from build123d import *

# Parameters (mm, degrees)
F0_R     = 4.1
F1_DEPTH = 3.4
F0_R_2   = 3.8
F0_R_3   = 1.95
F2_DEPTH = 3.72
F3_DEPTH = 3.28
F4_SIZE  = 0.1
F5_SIZE  = 0.1
F6_SIZE  = 0.1
F7_DEPTH = 3.72


# Not quite as in the source:
# - a feature names something its author has since deleted; it is built from what else it names


with BuildPart() as f1:
    # F0 (on Front) → F1 (new body)
    with BuildSketch(Plane.XZ):
        with BuildLine():
            ThreePointArc((-9.1306946704, 2.3368867827), (-8.1937279785, 1.5734002793), (-7.0529357563, 1.1741367966))
            ThreePointArc((-7.0529357563, 1.1741367966), (-7.1195743604, 0.6589088915), (-7.1486252748, 0.1402022865))
            ThreePointArc((-7.1486252748, 0.1402022865), (-8.3432287104, -0.042236429), (-9.4045806012, -0.6200715414))
            ThreePointArc((-9.4045806012, -0.6200715414), (-9.3954740629, -0.7454476061), (-9.384696163, -0.870691063))
            ThreePointArc((-9.384696163, -0.870691063), (-9.3722488189, -0.9957796327), (-9.3581342447, -1.120691063))
            ThreePointArc((-9.3581342447, -1.120691063), (-8.2085925976, -1.4934044314), (-7.0008156513, -1.4529556828))
            ThreePointArc((-7.0008156513, -1.4529556828), (-6.8768331336, -1.9574641892), (-6.7165444751, -2.4516382918))
            ThreePointArc((-6.7165444751, -2.4516382918), (-7.76441436, -3.053950319), (-8.544935067, -3.9767712658))
            ThreePointArc((-8.544935067, -3.9767712658), (-8.4914364249, -4.0897594601), (-8.43644384, -4.2020281216))
            ThreePointArc((-8.43644384, -4.2020281216), (-8.3799669873, -4.3135574983), (-8.3220158032, -4.4243279682))
            ThreePointArc((-8.3220158032, -4.4243279682), (-7.1152349462, -4.3573127689), (-6.0032028311, -3.8838197394))
            ThreePointArc((-6.0032028311, -3.8838197394), (-5.7053436074, -4.3094726268), (-5.3773631048, -4.7123737159))
            ThreePointArc((-5.3773631048, -4.7123737159), (-6.1368874979, -5.6525550384), (-6.5313316874, -6.7950225452))
            ThreePointArc((-6.5313316874, -6.7950225452), (-6.4406375804, -6.8810473446), (-6.3488105376, -6.9658617383))
            ThreePointArc((-6.3488105376, -6.9658617383), (-6.255866712, -7.0494508071), (-6.1618224526, -7.1317998474))
            ThreePointArc((-6.1618224526, -7.1317998474), (-5.0607335264, -6.6333809478), (-4.1948295471, -5.7901558762))
            ThreePointArc((-4.1948295471, -5.7901558762), (-3.7633208909, -6.0794667424), (-3.3119438366, -6.3366811521))
            ThreePointArc((-3.3119438366, -6.3366811521), (-3.6805479914, -7.487745529), (-3.6356508664, -8.6955544836))
            ThreePointArc((-3.6356508664, -8.6955544836), (-3.5200054468, -8.7430078723), (-3.4037408432, -8.7889233284))
            ThreePointArc((-3.4037408432, -8.7889233284), (-3.2868775071, -8.8332927753), (-3.1694359951, -8.8761084081))
            ThreePointArc((-3.1694359951, -8.8761084081), (-2.3227497605, -8.0135884705), (-1.8199250223, -6.9145045313))
            ThreePointArc((-1.8199250223, -6.9145045313), (-1.3130441845, -7.0284005982), (-0.7992311491, -7.1051903261))
            ThreePointArc((-0.7992311491, -7.1051903261), (-0.727143962, -8.311678782), (-0.2489808346, -9.4217107546))
            ThreePointArc((-0.2489808346, -9.4217107546), (-0.123991383, -9.4241843752), (0.0010198831, -9.4249999448))
            ThreePointArc((0.0010198831, -9.4249999448), (0.1260309698, -9.4241573201), (0.2510198831, -9.4216566494))
            ThreePointArc((0.2510198831, -9.4216566494), (0.7289427654, -8.3115212183), (0.8007688415, -7.1050171895))
            ThreePointArc((0.8007688415, -7.1050171895), (1.3145652461, -7.0281162635), (1.8214214224, -6.9141104997))
            ThreePointArc((1.8214214224, -6.9141104997), (2.3244840135, -8.0130855914), (3.1713568956, -8.8754222683))
            ThreePointArc((3.1713568956, -8.8754222683), (3.2887891386, -8.8325812196), (3.4056428696, -8.7881864821))
            ThreePointArc((3.4056428696, -8.7881864821), (3.5218975334, -8.742245865), (3.6375326803, -8.6947674494))
            ThreePointArc((3.6375326803, -8.6947674494), (3.6821684093, -7.4869488064), (3.3133151488, -6.3359642301))
            ThreePointArc((3.3133151488, -6.3359642301), (3.764636526, -6.078652139), (4.1960825592, -5.7892478921))
            ThreePointArc((4.1960825592, -5.7892478921), (5.0621690097, -6.6322855443), (6.1633657783, -7.1304661337))
            ThreePointArc((6.1633657783, -7.1304661337), (6.2573922134, -7.0480967422), (6.3503179465, -6.9644875604))
            ThreePointArc((6.3503179465, -6.9644875604), (6.4421266315, -6.8796532953), (6.5328021188, -6.7936088699))
            ThreePointArc((6.5328021188, -6.7936088699), (6.1381106848, -5.6512267557), (5.3783828347, -4.7112098322))
            ThreePointArc((5.3783828347, -4.7112098322), (5.7062761334, -4.3082377707), (6.00404323, -3.8825204303))
            ThreePointArc((6.00404323, -3.8825204303), (7.1161845365, -4.3557644871), (8.3229834462, -4.4225073832))
            ThreePointArc((8.3229834462, -4.4225073832), (8.3809053661, -4.3117340184), (8.4373530488, -4.2002022011))
            ThreePointArc((8.4373530488, -4.2002022011), (8.492316565, -4.0879315502), (8.5457862464, -3.9749418147))
            ThreePointArc((8.5457862464, -3.9749418147), (7.7650725635, -3.0522802473), (6.7170749034, -2.4501846343))
            ThreePointArc((6.7170749034, -2.4501846343), (6.8772566086, -1.9559758535), (7.0011299372, -1.4514405265))
            ThreePointArc((7.0011299372, -1.4514405265), (8.2090091905, -1.4913388042), (9.3584507476, -1.1180449923))
            ThreePointArc((9.3584507476, -1.1180449923), (9.3724970598, -0.9934404183), (9.3848843789, -0.868659999))
            ThreePointArc((9.3848843789, -0.868659999), (9.3956105125, -0.7437258211), (9.4046735619, -0.618659999))
            ThreePointArc((9.4046735619, -0.618659999), (8.3432765874, -0.0407321266), (7.1485947646, 0.1417493946))
            ThreePointArc((7.1485947646, 0.1417493946), (7.119431592, 0.6604497002), (7.0526814835, 1.1756631713))
            ThreePointArc((7.0526814835, 1.1756631713), (8.19338727, 1.5751735359), (9.1301887056, 2.3388628005))
            ThreePointArc((9.1301887056, 2.3388628005), (9.0983662855, 2.4597471284), (9.0649434237, 2.5801987762))
            ThreePointArc((9.0649434237, 2.5801987762), (9.0299259996, 2.7001965561), (8.9933201729, 2.8197193598))
            ThreePointArc((8.9933201729, 2.8197193598), (7.794773105, 2.9756140317), (6.6146636541, 2.7145395084))
            ThreePointArc((6.6146636541, 2.7145395084), (6.4000942258, 3.1876784501), (6.1517355927, 3.6439880896))
            ThreePointArc((6.1517355927, 3.6439880896), (7.0710932374, 4.4285897362), (7.6687594725, 5.4791197426))
            ThreePointArc((7.6687594725, 5.4791197426), (7.5954176181, 5.5803455276), (7.5207396972, 5.6805897059))
            ThreePointArc((7.5207396972, 5.6805897059), (7.444738846, 5.7798346442), (7.3674284334, 5.8780628849))
            ThreePointArc((7.3674284334, 5.8780628849), (6.1935005716, 5.5904666436), (5.1873914517, 4.9207184361))
            ThreePointArc((5.1873914517, 4.9207184361), (4.8163943669, 5.2843963991), (4.4199691978, 5.6201754679))
            ThreePointArc((4.4199691978, 5.6201754679), (4.9938151748, 6.683904295), (5.1716286044, 7.8793960795))
            ThreePointArc((5.1716286044, 7.8793960795), (5.0666724743, 7.9472923086), (4.9608250949, 8.0137905749))
            ThreePointArc((4.9608250949, 8.0137905749), (4.8541050851, 8.0788791811), (4.7465312174, 8.1425466779))
            ThreePointArc((4.7465312174, 8.1425466779), (3.7557669795, 7.4503007335), (3.0595379066, 6.4623314522))
            ThreePointArc((3.0595379066, 6.4623314522), (2.5822180472, 6.6674320361), (2.0912654051, 6.8373320093))
            ThreePointArc((2.0912654051, 6.8373320093), (2.2421089696, 8.0365222748), (1.9760667465, 9.2155187165))
            ThreePointArc((1.9760667465, 9.2155187165), (1.8536604305, 9.2409181367), (1.7309279903, 9.2646917538))
            ThreePointArc((1.7309279903, 9.2646917538), (1.6078910188, 9.2868353852), (1.4845711627, 9.307345135))
            ThreePointArc((1.4845711627, 9.307345135), (0.8107889051, 8.3039366723), (0.5184795371, 7.1311765488))
            ThreePointArc((0.5184795371, 7.1311765488), (-0.0006988298, 7.1499999658), (-0.5198735073, 7.1310750618))
            ThreePointArc((-0.5198735073, 7.1310750618), (-0.8124228005, 8.3037784061), (-1.4864122256, 9.307051289))
            ThreePointArc((-1.4864122256, 9.307051289), (-1.609717186, 9.2865190239), (-1.7327389902, 9.2643532204))
            ThreePointArc((-1.7327389902, 9.2643532204), (-1.8554559982, 9.2405577775), (-1.9778466235, 9.2151368809))
            ThreePointArc((-1.9778466235, 9.2151368809), (-2.2436700583, 8.0360880591), (-2.0926019054, 6.8369230846))
            ThreePointArc((-2.0926019054, 6.8369230846), (-2.5835911424, 6.6669000899), (-3.0609364181, 6.4616691531))
            ThreePointArc((-3.0609364181, 6.4616691531), (-3.7573792917, 7.4494877329), (-4.7482933229, 8.141519239))
            ThreePointArc((-4.7482933229, 8.141519239), (-4.8558534091, 8.0778284625), (-4.9625593299, 8.0127167613))
            ThreePointArc((-4.9625593299, 8.0127167613), (-5.0683923152, 7.946195589), (-5.1733337487, 7.8782766469))
            ThreePointArc((-5.1733337487, 7.8782766469), (-4.9952615939, 6.6828233728), (-4.4211854174, 5.6192187629))
            ThreePointArc((-4.4211854174, 5.6192187629), (-4.8175379075, 5.2833539073), (-5.1884562761, 4.9195956613))
            ThreePointArc((-5.1884562761, 4.9195956613), (-6.19471032, 5.5891261102), (-7.3687003961, 5.8764682823))
            ThreePointArc((-7.3687003961, 5.8764682823), (-7.4459895483, 5.7782233123), (-7.521968919, 5.6789619282))
            ThreePointArc((-7.521968919, 5.6789619282), (-7.5966251432, 5.5787015903), (-7.6699450885, 5.477459935))
            ThreePointArc((-7.6699450885, 5.477459935), (-7.0720515108, 4.4270593007), (-6.1525240836, 3.6426566406))
            ThreePointArc((-6.1525240836, 3.6426566406), (-6.4007839559, 3.1862932618), (-6.6152509821, 2.7131078939))
            ThreePointArc((-6.6152509821, 2.7131078939), (-7.7954169073, 2.9739270108), (-8.9939302083, 2.817772952))
            ThreePointArc((-8.9939302083, 2.817772952), (-9.0305101669, 2.6982422288), (-9.0655016202, 2.5782368733))
            ThreePointArc((-9.0655016202, 2.5782368733), (-9.0988984129, 2.4577779948), (-9.1306946704, 2.3368867827))
        make_face()
        Circle(F0_R, mode=Mode.SUBTRACT)
    extrude(amount=F1_DEPTH)



with BuildPart() as f2:
    # F0 (on Front) → F2 (new body)
    with BuildSketch(Plane.XZ):
        Circle(F0_R_2)
        Circle(F0_R_3, mode=Mode.SUBTRACT)
    extrude(amount=F2_DEPTH)

    # F0 (on Front) → F3 (join)
    with BuildSketch(Plane.XZ):
        Circle(F0_R_2)
        Circle(F0_R_3, mode=Mode.SUBTRACT)
    extrude(amount=-F3_DEPTH)

    # F4
    f4_edges = [f2.edges().sort_by_distance(p)[0] for p in [
        (-1.95, 3.28, 0),
    ]]
    chamfer(f4_edges, length=F4_SIZE)

    # F5
    f5_edges = [f2.edges().sort_by_distance(p)[0] for p in [
        (-1.95, -3.72, 0),
    ]]
    chamfer(f5_edges, length=F5_SIZE)

    # F6
    f6_edges = [f2.edges().sort_by_distance(p)[0] for p in [
        (-3.8, 3.28, 0),
    ]]
    chamfer(f6_edges, length=F6_SIZE)


with BuildPart() as f1_1:
    add(f1.part)

    add(f2.part)  # F7 merges F2
    # F0 (on Front) → F7 (join)
    with BuildSketch(Plane.XZ):
        Circle(F0_R)
        Circle(F0_R_2, mode=Mode.SUBTRACT)
    extrude(amount=F7_DEPTH)


solid = f1_1.part
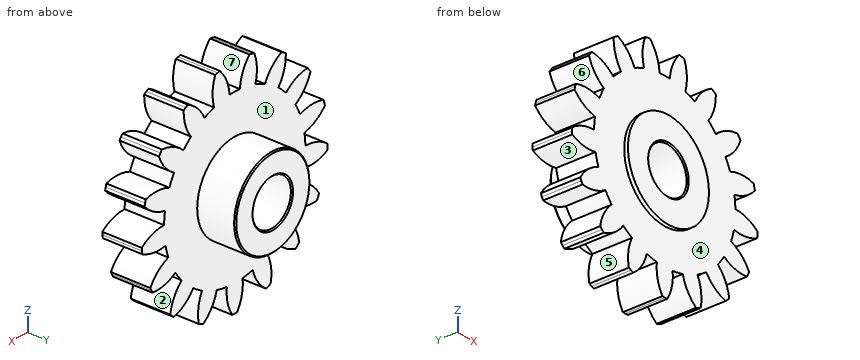
Source: CAD feature listing. Evaluate the final solid. Frame: model axes, mm. Face numbers are marked on the shaded views. A direction names the side the tool comes from. Round coordinates to 2 decimals unless told otherwise and drop trailing zeros. Loops run counter-clockwise (first coordinate to the right, second up) from the corner with the lowest first, then second, coordinate; pieces in that order, holes last. Notation, with made-up numbers: M -3.5,-10 L 0.5,-10 A14 cw 0.5,15 Z; hole C -30,11.5 d8. An arc over 180 degrees is marked long. Return JSON: item names as keys, results as strings. Group by question number.
1. Reachability of the marked faces 4, 5, 6 and 7 from +Z, -Z, +X, -X, +Y, -Y: full face, straight path, thin tool, end or side. Return the list, or none.
2. Pin query (flat end, axial travel): pin 1 (4 mm diameter, centred on x = 1, y = 2.5, fed in from +Z); pin 2 (1 mm diameter, centred on x = -6, z = -6, fed in from -Y); pin 3 (2 mm diameter, centred on x = -5, z = -5.5, fed in from +Y). Return the tip coordinate at first contact, or that it passes through.
3. Mould query, pull axis X, two halves, no side actions, for the marked faces 1, 2 and 3. Classes: released by +X, released by -X, zero draft, split by the parting line, or undercut.
4. Section query A-A on x = -5.75. Output: boundary loops of the cut face in (y, z).
5. Section query B-B on y = 1. Output: boundary loops of the cut face in (x, z).
6. Material intervals for line 1 along X through (y, z) = (-2.75, -8); line 2 along X through (y, z) = (-1, -7.25); line 3 along Z through (x, y) = (0, -0.25) (3 decimals), sorted ascending. Write a range as from..to.
7. Section query C-C on z = -5.25. Output: boundary loops of the cut face in (x, y).
Checks:
{
 "1": {"face 4": "-Y", "face 5": "+Y, -Y", "face 6": "-X, +Y, -Y", "face 7": "+Z, +Y, -Y"},
 "2": {"pin 1": "stops at z = 3.8", "pin 2": "stops at y = -3.4", "pin 3": "stops at y = 0"},
 "3": {"face 1": "zero draft", "face 2": "released by +X", "face 3": "undercut"},
 "4": {"outline": "M -3.4,-7 L 0,-7 L 0,-5.09 L -3.4,-5.09 Z; M -3.4,-4.25 L 0,-4.25 L 0,5.35 L -3.4,5.35 Z"},
 "5": {"outline": "C 0,0 d7.6; hole C 0,0 d3.9"},
 "6": {"line 1": "x = -3.71..-2.31, -0.79..0.79, 2.32..3.71", "line 2": "x = -3.64..-1.93, -0.81..0.81, 1.93..3.64", "line 3": "z = -9.425..-1.95, 1.95..7.15"},
 "7": {"outline": "M -5.88,-3.4 L 5.88,-3.4 L 5.88,0 L -5.88,0 Z"}
}
